```python
from build123d import *

# Parameters (mm, degrees)
SKETCH1_W               = 63.5
SKETCH1_H               = 57.15
BOSS_EXTRUDE1_DEPTH     = 12.7
SKETCH2_W               = 63.5
SKETCH2_H               = 19.05
CUT_EXTRUDE1_DEPTH      = 6.35
F_3_8_CLEARANCE_HOLE1_D = 10.0838
SKETCH10_W              = 63.5
SKETCH10_H              = 12.7
BOSS_EXTRUDE2_DEPTH     = 63.5
SKETCH11_W              = 19.05
SKETCH11_H              = 60.325
CUT_EXTRUDE3_DEPTH      = 6.35
FILLET1_R               = 4.7625
F_1_4_CLEARANCE_HOLE1_D = 6.7564
SKETCH13_W              = 19.05
SKETCH13_H              = 63.5
CUT_EXTRUDE5_DEPTH      = 99.219947694
FILLET2_R               = 9.525
F_10_24_TAPPED_HOLE1_D  = 3.7973


with BuildPart() as part:
    # Sketch1 → Boss-Extrude1 (new body)
    with BuildSketch(Plane(origin=(0, 0, 0), x_dir=(1, 0, 0), z_dir=(0, 1, 0))):
        Rectangle(SKETCH1_W, SKETCH1_H)
    extrude(amount=BOSS_EXTRUDE1_DEPTH)

    # Sketch2 → Cut-Extrude1 (cut)
    with BuildSketch(Plane.XZ):
        Rectangle(SKETCH2_W, SKETCH2_H)
    extrude(amount=-CUT_EXTRUDE1_DEPTH, mode=Mode.SUBTRACT)

    # 3/8 Clearance Hole1 (through all)
    with Locations(Plane(origin=(0, 12.7, 0), x_dir=(1, 0, 0), z_dir=(0, 1, 0))):
        with Locations((-9.525, 19.05), (-9.525, -19.05)):
            Hole(F_3_8_CLEARANCE_HOLE1_D / 2)

    # Sketch10 → Boss-Extrude2 (add)
    with BuildSketch(Plane(origin=(0, 0, -28.575), x_dir=(-1, 0, 0), z_dir=(0, 0, -1))):
        with Locations((0, 6.35)):
            Rectangle(SKETCH10_W, SKETCH10_H)
    extrude(amount=BOSS_EXTRUDE2_DEPTH)

    # Sketch11 → Cut-Extrude3 (cut)
    with BuildSketch(Plane.XZ):
        with Locations((-9.525, -61.9125)):
            Rectangle(SKETCH11_W, SKETCH11_H)
    extrude(amount=-CUT_EXTRUDE3_DEPTH, mode=Mode.SUBTRACT)

    # Fillet1
    fillet1_edges = [part.edges().sort_by_distance(p)[0] for p in [
        (0, 3.175, -31.75),
        (-19.05, 3.175, -31.75),
    ]]
    fillet(fillet1_edges, radius=FILLET1_R)

    # 1/4 Clearance Hole1 (through all)
    with Locations(Plane(origin=(0, 6.35, 0), x_dir=(-1, 0, 0), z_dir=(0, -1, 0))):
        with Locations((-22.225, 0), (9.525, 49.2125)):
            Hole(F_1_4_CLEARANCE_HOLE1_D / 2)

    # Sketch13 → Cut-Extrude5 (cut, through all)
    with BuildSketch(Plane.XZ):
        with Locations((22.225, -60.325)):
            Rectangle(SKETCH13_W, SKETCH13_H)
    extrude(amount=-CUT_EXTRUDE5_DEPTH, mode=Mode.SUBTRACT)

    # Fillet2
    fillet2_edges = [part.edges().sort_by_distance(p)[0] for p in [
        (12.7, 6.35, -28.575),
    ]]
    fillet(fillet2_edges, radius=FILLET2_R)

    # #10-24 Tapped Hole1 (through all)
    with Locations(Plane(origin=(0, 12.7, 0), x_dir=(1, 0, 0), z_dir=(0, 1, 0))):
        with Locations((19.05, 19.05)):
            Hole(F_10_24_TAPPED_HOLE1_D / 2)


solid = part.part
```
Input: part model. Units: mm. Frame: model coordinates. A direction names the side the tool comes from. Give positions to 0.01 mm unless a question says otherwise; leave off trailing zeros. Write each loop counter-clockwise with the first axis right and the second up, starting at its lowest first coordinate (ties: lowest second). Pieces come first, ordered by that corner, then holes. Notation, with made-up numbers: (41, -8.5) - (98, -8.5) arc R28 ccw to (98, 11.5) - close; hole circle Ø1 at (62, 86.5). An arc over 180 degrees is marked (long way). Write item = value, one per line. Start each with the question number.
1) Cut plane B-B (z = -19.05). Return loops of the section in (x, y).
2) Material intervals for L1, parallel to X at y = 10.25, z = -19.05; L2, parallel to Z at x = 1.5, y = 6 (3 decimals); L3, parallel to X at y = 0.75, z = -55, sorted ascending. Write a range as [from, to].
3) Reachability of faces 1 (the face through (0, 3, -9.525)), 2 (the face through (-8.87, 6.26, -24.05)), 3 (the face through (-19.05, 3, -65)) from +Z, -Z, +X, -X, +Y, -Y: full face, straight path, thin tool, end or side. Return the list, or none.
4) Cut plane D-D (x = -10.5). Return loops of the section in (y, z) (3 decimals), and give its area (3 significant figures).
5) Cut plane C-C (z = 0). Return loops of the section in (x, y).
6) Cut plane A-A (y = 1.5). Give the number of separate pieces and of enclosed holes in the cut face, and give its area (3 significant figures).
7) Draft query along Z for faces 4 (the face through (-9.965, 9.569, -52.562)), 5 (the face through (-10, 3, -31.75)), 6 (the face through (12.7, 6, -65)), 7 (the face through (0, 3, 9.525)). Return one class per face: pulls with the +Z half, pulls with the -Z half, needs draft (parallel to the pull), parting line crosses it, or undercut.
8) Pin query (flat end, axial travel): pin 1 (5.5 mm diameter, centred on x = -12.5, z = -58, fed in from -Y); pin 2 (7 mm diameter, centred on x = -9, y = 2.5, fed in from -Z); pin 3 (5 mm diameter, centred on x = 13.5, y = 8.5, fed in from -Z) (3 decimals); pin 4 (7 mm diameter, centred on y = 4.5, z = -61, fed in from +X). Return the tip coordinate at first contact, or that it passes through.
Answers follow:
q1.outline = (-31.75, 0) - (-14.57, 0) - (-14.57, 12.7) - (-31.75, 12.7) - close; (-4.48, 0) - (17.15, 0) - (17.15, 12.7) - (-4.48, 12.7) - close; (20.95, 0) - (31.75, 0) - (31.75, 12.7) - (20.95, 12.7) - close
q2.L1 = [-31.75, -14.57], [-4.48, 17.15], [20.95, 31.75]
q2.L2 = [-92.075, -9.525], [9.525, 28.575]
q2.L3 = [-31.75, -19.05], [0, 12.7]
q3.face_1 = +X, -X, -Y
q3.face_2 = +Y, -Y
q3.face_3 = -Z, -Y
q4.outline = (0, -31.75) - (6.35, -31.75) - (6.35, -45.978) - (12.7, -45.978) - (12.7, -23.997) - (0, -23.997) - close; (0, -14.103) - (12.7, -14.103) - (12.7, 14.103) - (0, 14.103) - (0, 9.525) - (6.35, 9.525) - (6.35, -9.525) - (0, -9.525) - close; (0, 23.997) - (12.7, 23.997) - (12.7, 28.575) - (0, 28.575) - close; (6.35, -92.075) - (12.7, -92.075) - (12.7, -52.447) - (6.35, -52.447) - close
q4.area = 736 mm^2
q5.outline = (-31.75, 6.35) - (18.85, 6.35) - (18.85, 12.7) - (-31.75, 12.7) - close; (25.6, 6.35) - (31.75, 6.35) - (31.75, 12.7) - (25.6, 12.7) - close
q6.separate_pieces = 2
q6.enclosed_holes = 3
q6.area = 3,950 mm^2
q7.face_4 = undercut
q7.face_5 = pulls with the -Z half
q7.face_6 = needs draft
q7.face_7 = undercut
q8.pin_1 = 6.35
q8.pin_2 = -31.75
q8.pin_3 = -92.075
q8.pin_4 = 12.7
